Source: CAD feature listing. Evaluate the final solid. Frame: model axes, mm. A direction names the side the tool comes from. Give positions to 0.01 mm unless a question says otherwise; leave off trailing zeros. Loops run counter-clockwise (first coordinate to the right, second up) from the corner with the lowest first, then second, coordinate; pieces in that order, holes last. Notation, with made-up numbers: M 6.5,52.5 L 22.5,52.5 A17 ccw 22.5,77.5 Z; hole C 2.5,0.5 d11. An arc over 180 degrees is marked long. Answer in a Markdown table with one row per item.
Autodesk Inventor part; units mm, degrees
ref_plane "YZ Plane" through (0, 0, 0) normal (1, 0, 0) x (0, 1, 0)
ref_plane "XZ Plane" through (0, 0, 0) normal (0, 1, 0) x (-1, 0, 0)
ref_plane "XY Plane" through (0, 0, 0) normal (0, 0, 1) x (1, 0, 0)
sketch "スケッチ1" plane through (0, 0, 0) normal (0, 0, 1) x (1, 0, 0)
  line L0 (0, 0) -> (5, 0)
  line L1 (5, 0) -> (5, 30)
  line L2 (5, 30) -> (0, 30)
  line L3 (0, 30) -> (0, 0)
  line L4 (5, 30) -> (15, 30)
  line L5 (15, 30) -> (15, 0)
  line L6 (15, 0) -> (5, 0)
  line L7 (5, 0) -> (5, 30)
  dimension "d0" = 30
  dimension "d1" = 5
  dimension "d2" = 30
  dimension "d3" = 10
extrude "押し出し1" add sketch "スケッチ1" along normal blind 5
sketch "スケッチ2" plane through (0, 0, 5) normal (0, 0, 1) x (1, 0, 0)
  line L0 (15, 0) -> (15, 30)
  line L1 (0, 0) -> (15, 0)
  line L2 (15, 30) -> (5, 30)
  line L3 (5, 30) -> (5, 0)
  line L4 (5, 0) -> (15, 0)
  line L5 (15, 0) -> (15, 30)
  point P0 (10, 21)
  point P1 (10, 9)
  dimension "d6" = 10
  dimension "d7" = 5
  dimension "d8" = 9
  dimension "d9" = 9
  dimension "d10" = 5
hole "穴1" at (10, 21, 5) at (10, 9, 5) direction (0, 0, -1) diameter 5 depth 8
sketch "スケッチ3" plane through (0, 0, 5) normal (0, 0, 1) x (1, 0, 0)
  line L0 (15, 30) -> (0, 30)
  line L1 (0, 0) -> (15, 0)
  line L2 (0, 30) -> (5, 30)
  line L3 (5, 30) -> (5, 0)
  line L4 (5, 0) -> (0, 0)
  line L5 (0, 0) -> (0, 30)
  dimension "d18" = 5
extrude "押し出し2" add sketch "スケッチ3" along normal blind 30
sketch "スケッチ4" plane through (5, 0, 5) normal (1, 0, 0) x (0, 0, -1)
  line L0 (-30, 0) -> (-30, 30)
  line L1 (0, 0) -> (-30, 0)
  line L2 (5, 0) -> (5, 30)
  point P0 (-20, 5)
  point P1 (-5, 5)
  dimension "d21" = 15
  dimension "d22" = 10
  dimension "d23" = 5
  dimension "d24" = 5
  dimension "d25" = 10
hole "穴2" at (5, 5, 25) at (5, 5, 10) direction (-1, 0, 0) diameter 5 depth 8
sketch "スケッチ5" plane through (5, 0, 5) normal (1, 0, 0) x (0, 0, -1)
  line L0 (5, 30) -> (-30, 30)
  line L1 (-30, 30) -> (-25, 30)
  line L2 (-25, 30) -> (-25, 0)
  line L3 (-25, 0) -> (-30, 0)
  line L4 (-30, 0) -> (-30, 30)
  line L5 (0, 0) -> (0, 30)
  circle A0 centre (-5, 5) radius 2.5
  circle A1 centre (-20, 5) radius 2.5
  point P0 (5, 0)
  dimension "d33" = 5
  dimension "d34" = 5
extrude "押し出し3" cut sketch "スケッチ5" against normal through all contours L2 L3 L4 L0
fillet "フィレット1" radius 2 4 edges at (2.5, 30, 30) (2.5, 0, 30) (15, 30, 2.5) (15, 0, 2.5)
fillet "フィレット2" radius 1 2 edges at (0, 15, 0) (5, 15, 5)
equation "\"d34\" = d33"
properties part number "BP_BOX-Support-Bar-Connect1"
1) Section A-A, the plane x = 10. Return loops of the section in (y, z).
Reply:
| item | result |
|---|---|
| outline | M 0,0 L 6.5,0 L 6.5,5 L 0,5 Z; M 11.5,0 L 18.5,0 L 18.5,5 L 11.5,5 Z; M 23.5,0 L 30,0 L 30,5 L 23.5,5 Z |
2) Section B-B, the plane y = 21. Return loops of the section in (x, z), then the cut area to 3 significant figures.
Reply:
| item | result |
|---|---|
| outline | M 0,1 A1 ccw 1,0 L 7.5,0 L 7.5,5 L 6,5 A1 cw 5,6 L 5,30 L 0,30 Z; M 12.5,0 L 15,0 L 15,5 L 12.5,5 Z |
| area | 175 mm² |
3) Section C-C, the plane z = 25. Return loops of the section in (x, y).
Reply:
| item | result |
|---|---|
| outline | M 0,0 L 5,0 L 5,2.5 L 0,2.5 Z; M 0,7.5 L 5,7.5 L 5,30 L 0,30 Z |
4) Pull-direction query (X, two-part tool) for faces 3 (the cylindrical face through (11.5, 23, 2.5)), 4 (the cylindrical face through (2.46, 29.4, 29.43)), 5 (the flat face through (0, 15, 15)), 6 (the cylindrical face through (12.44, 9.54, 2.46)); classes: released by +X, released by -X, zero draft, split by the parting line, or undercut.
Reply:
| item | result |
|---|---|
| face 3 | undercut |
| face 4 | zero draft |
| face 5 | released by -X |
| face 6 | undercut |
5) Material intervals for L1, parallel to Y at x = 10, z = 3.2; L2, parallel to X at y = 21, z = 2.35; L3, parallel to Z at x = 3.7, y = 5, sorted ascending.
Reply:
| item | result |
|---|---|
| L1 | y = 0 to 6.5, 11.5 to 18.5, 23.5 to 30 |
| L2 | x = 0 to 7.5, 12.5 to 15 |
| L3 | z = 0 to 7.5, 12.5 to 22.5, 27.5 to 30 |
6) Pin query (flat end, axial travel): pin 1 Ø2 at (x, y) = (9, 25.5) entering from +Z. Return the tip coordinate at first contact, or that it passes through.
Reply:
| item | result |
|---|---|
| pin 1 | stops at z = 5 |
7) Set-up query: faces 1 (the flat face through (3, 15, 30)), 2 (the flat face through (5, 15, 18)). Return all of +Z, -Z, +X, -X, +Y, -Y with unobstructed straight access to the full face (end or side cutting, diameter ignored); none if empty.
Reply:
| item | result |
|---|---|
| face 1 | +Z, +X, -X, +Y, -Y |
| face 2 | +Z, +X, +Y, -Y |
8) Section D-D, the plane y = 5. Return loops of the section in (x, z).
Reply:
| item | result |
|---|---|
| outline | M 0,1 A1 ccw 1,0 L 15,0 L 15,5 L 6,5 A1 cw 5,6 L 5,7.5 L 0,7.5 Z; M 0,12.5 L 5,12.5 L 5,22.5 L 0,22.5 Z; M 0,27.5 L 5,27.5 L 5,30 L 0,30 Z |
